from build123d import *

# Parameters (mm, degrees)
SKETCH_1_R        = 20
EXTRUDE_1_DEPTH   = 6
HOLE_WIZARD_M31_D = 2.5


with BuildPart() as part:
    # Эскиз1 → Бобышка-Вытянуть1 (new body)
    with BuildSketch(Plane.XY):
        with BuildLine():
            Line((9.476919675, -23.134130489), (21.23028272, -25.76965455))
            ThreePointArc((21.23028272, -25.76965455), (24.748737342, -24.748737342), (25.76965455, -21.23028272))
            Line((25.76965455, -21.23028272), (23.134130489, -9.476919675))
            ThreePointArc((23.134130489, -9.476919675), (17.67766953, 17.67766953), (-9.476919675, 23.134130489))
            Line((-9.476919675, 23.134130489), (-21.23028272, 25.76965455))
            ThreePointArc((-21.23028272, 25.76965455), (-24.748737342, 24.748737342), (-25.76965455, 21.23028272))
            Line((-25.76965455, 21.23028272), (-23.134130489, 9.476919675))
            ThreePointArc((-23.134130489, 9.476919675), (-17.67766953, -17.67766953), (9.476919675, -23.134130489))
        make_face()
        Circle(SKETCH_1_R, mode=Mode.SUBTRACT)
    extrude(amount=EXTRUDE_1_DEPTH)

    # Отверстие обработанное метчиком M31 (through all)
    with Locations(Plane.XY.offset(6)):
        with Locations((-22.061731573, 22.061731573), (22.061731573, -22.061731573)):
            Hole(HOLE_WIZARD_M31_D / 2)


solid = part.part
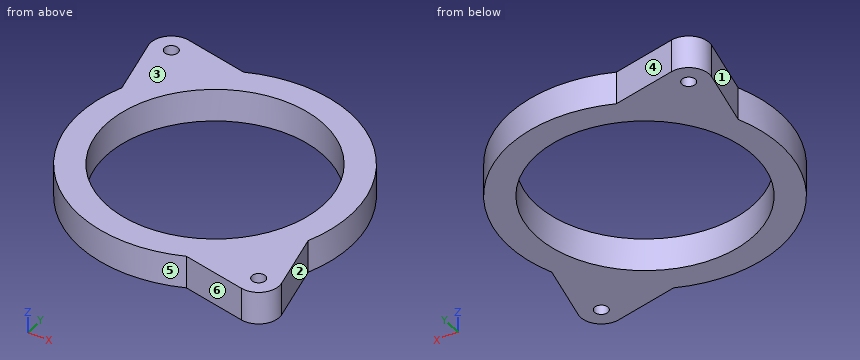
Source: CAD feature listing. Evaluate the final solid. Frame: model axes, mm. Face numbers are marked on the shaded views. A direction names the side the tool comes from. Round coordinates to 2 decimals unless told otherwise and drop trailing zeros. Loops run counter-clockwise (first coordinate to the right, second up) from the corner with the lowest first, then second, coordinate; pieces in that order, holes last. Notation, with made-up numbers: M 72.25,51.5 L 126.25,51.5 A9 ccw 126.25,66.5 Z; hole C -23,-1 d5. An arc over 180 degrees is marked long. Return JSON: item names as keys, results as strings. Group by question number.
1. Material intervals for line 1 along Y through (x, z) = (0.5, 1.45) (3 decimals); line 2 along X through (y, z) = (-11.5, 4.1); line 3 along Y through (x, z) = (2, 3.85), sorted ascending. Write a range as from..to.
2. Mould query, pull axis Y, two halves, no side actions, for the marked faces 4, 5 and 6. Classes: released by +Y, released by -Y, zero draft, split by the parting line, or undercut.
3. Section query C-C on z = 5.1. Output: boundary loops of the cut face in (x, y), and give its area (3 significant figures).
4. Pin query (flat end, axial travel): pin 1 (1 mm diameter, centred on x = 0.5, z = 2.5, fed in from +Y); pin 2 (1 mm diameter, centred on y = -17, z = 2.5, fed in from +X); pin 3 (2 mm diameter, centred on y = -11.5, z = 3, fed in from +X). Return the tip coordinate at first contact, or that it passes through.
5. Reachability of the marked faces 1, 2 and 3 from +Z, -Z, +X, -X, +Y, -Y: full face, straight path, thin tool, end or side. Return the list, or none.
6. Section query A-A on y = 0. Output: boundary loops of the cut face in (x, z).
Checks:
{
 "1": {"line 1": "y = -24.995..-19.994, 19.994..24.995", "line 2": "x = -22.2..-16.36, 16.36..23.59", "line 3": "y = -24.92..-19.9, 19.9..24.92"},
 "2": {"face 4": "released by +Y", "face 5": "undercut", "face 6": "released by -Y"},
 "3": {"outline": "M -25.77,21.23 L -23.13,9.48 A25 ccw 9.48,-23.13 L 21.23,-25.77 A3.8 ccw 25.77,-21.23 L 23.13,-9.48 A25 ccw -9.48,23.13 L -21.23,25.77 A3.8 ccw Z; hole C -22.06,22.06 d2.5; hole C 0,0 d40; hole C 22.06,-22.06 d2.5", "area": "924 mm²"},
 "4": {"pin 1": "stops at y = 25", "pin 2": "stops at x = 24.93", "pin 3": "stops at x = 23.81"},
 "5": {"face 1": "+Z, -Z, -X", "face 2": "+Z, -Z, +X", "face 3": "+Z, +X, -X, +Y, -Y"},
 "6": {"outline": "M -25,0 L -20,0 L -20,6 L -25,6 Z; M 20,0 L 25,0 L 25,6 L 20,6 Z"}
}
